For this review, take the finished solid that the model builds, in its own axes (mm). A direction names the side the tool comes from. Round coordinates to 2 decimals unless told otherwise and drop trailing zeros. Write each loop counter-clockwise with the first axis right and the second up, starting at its lowest first coordinate (ties: lowest second). Pieces come first, ordered by that corner, then holes. Notation, with made-up numbers: M 89,-37 L 94,-37 A28 cw 94,-14 Z; hole C 77,18 d7. An arc over 180 degrees is marked long. Answer in a Markdown table with one row per item.
Autodesk Inventor part; units mm, degrees
ref_plane "YZ Plane" through (0, 0, 0) normal (1, 0, 0) x (0, 1, 0)
ref_plane "XZ Plane" through (0, 0, 0) normal (0, 1, 0) x (-1, 0, 0)
ref_plane "XY Plane" through (0, 0, 0) normal (0, 0, 1) x (1, 0, 0)
sketch "Esquisse1" plane through (0, 0, 0) normal (0, 0, 1) x (1, 0, 0)
  line L0 (0, 16) -> (41, 16)
  line L1 (41, 16) -> (41, 0)
  line L2 (41, 0) -> (0, 0)
  line L3 (0, 0) -> (0, 16)
  line L4 (0, -3.2) -> (0, 19.2)
  line L5 (-8.2, 0) -> (49.2, 0)
  point P0 (0, 0)
  dimension "d0" = 16
  dimension "d1" = 41
extrude "Extrusion1" add sketch "Esquisse1" along normal blind 2
sketch "Esquisse2" plane through (0, 0, 2) normal (0, 0, 1) x (1, 0, 0)
  line L0 (1, 13) -> (3.5, 13)
  line L1 (3.5, 13) -> (3.5, 10.5)
  line L2 (3.5, 10.5) -> (1, 10.5)
  line L3 (1, 10.5) -> (1, 13)
  line L4 (3.5, 13) -> (6, 13)
  line L5 (6, 13) -> (6, 10.5)
  line L6 (6, 10.5) -> (3.5, 10.5)
  line L7 (3.5, 10.5) -> (3.5, 13)
  line L8 (0, -3.2) -> (0, 19.2)
  line L9 (1, 8) -> (1, 10.5)
  line L10 (1, 10.5) -> (3.5, 10.5)
  line L11 (3.5, 10.5) -> (3.5, 8)
  line L12 (3.5, 10.5) -> (6, 10.5)
  line L13 (6, 10.5) -> (6, 8)
  line L14 (6, 8) -> (3.5, 8)
  line L15 (3.5, 8) -> (1, 8)
  line L16 (1, 5.5) -> (1, 8)
  line L17 (1, 8) -> (3.5, 8)
  line L18 (3.5, 8) -> (3.5, 5.5)
  line L19 (3.5, 8) -> (6, 8)
  line L20 (6, 8) -> (6, 5.5)
  line L21 (6, 5.5) -> (3.5, 5.5)
  line L22 (3.5, 5.5) -> (1, 5.5)
  line L23 (1, 3) -> (1, 5.5)
  line L24 (1, 5.5) -> (3.5, 5.5)
  line L25 (3.5, 5.5) -> (3.5, 3)
  line L26 (3.5, 5.5) -> (6, 5.5)
  line L27 (6, 5.5) -> (6, 3)
  line L28 (6, 3) -> (3.5, 3)
  line L29 (3.5, 3) -> (1, 3)
  line L30 (41, 16) -> (0, 16)
  point P0 (0, 0)
  dimension "d4" = 2.5
  dimension "d5" = 2.5
  dimension "d8" = 2.5
  dimension "d9" = 2.5
  dimension "d12" = 2.5
  dimension "d17" = 3
  dimension "d18" = 1
extrude "Extrusion2" add sketch "Esquisse2" along normal blind 2
sketch "Esquisse3" plane through (0, 0, 4) normal (0, 0, 1) x (1, 0, 0)
  line L0 (1.85, 12.15) -> (2.65, 12.15)
  line L1 (2.65, 12.15) -> (2.65, 11.35)
  line L2 (2.65, 11.35) -> (1.85, 11.35)
  line L3 (1.85, 11.35) -> (1.85, 12.15)
  line L4 (6, 13) -> (1, 13)
  line L5 (1, 13) -> (1, 3)
  line L6 (2.65, 9.65) -> (2.65, 8.85)
  line L7 (1.85, 9.65) -> (2.65, 9.65)
  line L8 (1.85, 8.85) -> (1.85, 9.65)
  line L9 (2.65, 8.85) -> (1.85, 8.85)
  line L10 (2.65, 7.15) -> (2.65, 6.35)
  line L11 (1.85, 7.15) -> (2.65, 7.15)
  line L12 (1.85, 6.35) -> (1.85, 7.15)
  line L13 (2.65, 6.35) -> (1.85, 6.35)
  line L14 (2.65, 4.65) -> (2.65, 3.85)
  line L15 (1.85, 4.65) -> (2.65, 4.65)
  line L16 (1.85, 3.85) -> (1.85, 4.65)
  line L17 (2.65, 3.85) -> (1.85, 3.85)
  line L18 (5.15, 12.15) -> (5.15, 11.35)
  line L19 (4.35, 12.15) -> (5.15, 12.15)
  line L20 (4.35, 11.35) -> (4.35, 12.15)
  line L21 (5.15, 11.35) -> (4.35, 11.35)
  line L22 (5.15, 9.65) -> (5.15, 8.85)
  line L23 (4.35, 9.65) -> (5.15, 9.65)
  line L24 (4.35, 8.85) -> (4.35, 9.65)
  line L25 (5.15, 8.85) -> (4.35, 8.85)
  line L26 (5.15, 7.15) -> (5.15, 6.35)
  line L27 (4.35, 7.15) -> (5.15, 7.15)
  line L28 (4.35, 6.35) -> (4.35, 7.15)
  line L29 (5.15, 6.35) -> (4.35, 6.35)
  line L30 (5.15, 4.65) -> (5.15, 3.85)
  line L31 (4.35, 4.65) -> (5.15, 4.65)
  line L32 (4.35, 3.85) -> (4.35, 4.65)
  line L33 (5.15, 3.85) -> (4.35, 3.85)
  point P0 (0, 0)
  dimension "d21" = 0.8
  dimension "d22" = 0.8
  dimension "d23" = 0.85
  dimension "d24" = 0.85
  dimension "d27" = 2.5
  dimension "d30" = 2.5
extrude "Extrusion3" add sketch "Esquisse3" along normal blind 6
sketch "Esquisse4" plane through (0, 0, 0) normal (0, 0, -1) x (-1, 0, 0)
  line L0 (-40, 5) -> (-34, 5)
  line L1 (-34, 5) -> (-34, 11)
  line L2 (-34, 11) -> (-40, 11)
  line L3 (-40, 11) -> (-40, 5)
  line L4 (-41, 0) -> (-41, 16)
  line L5 (0, 0) -> (-41, 0)
  dimension "d35" = 6
  dimension "d36" = 6
  dimension "d37" = 1
  dimension "d38" = 5
extrude "Extrusion4" add sketch "Esquisse4" along normal blind 3
sketch "Esquisse5" plane through (0, 0, -3) normal (0, 0, -1) x (-1, 0, 0)
  circle A0 centre (-37, 8) radius 3
  line L0 (-34, 11) -> (-40, 11)
  line L1 (-40, 11) -> (-40, 5)
  line L2 (-34, 5) -> (-34, 11)
  point P0 (0, 0)
extrude "Extrusion5" add sketch "Esquisse5" along normal blind 1 contours A0
sketch "Esquisse6" plane through (37, 8, -4) normal (0, 0, -1) x (-1, 0, 0)
  line L0 (-3, -3) -> (3, -3)
  line L1 (3, -3) -> (3, 3)
  line L2 (3, 3) -> (-3, 3)
  line L3 (-3, 3) -> (-3, -3)
  line L4 (0, 3) -> (-3, 3)
  line L5 (-3, 0) -> (-3, -3)
  line L6 (-3, -3) -> (0, -3)
  line L7 (3, -3) -> (3, 0)
  point P0 (37, -8)
extrude "Extrusion6" add sketch "Esquisse6" along normal blind 7
sketch "Esquisse7" plane through (40, 8, -4) normal (1, 0, 0) x (0, 0, -1)
  circle A0 centre (4, 0) radius 3
  line L0 (7, 3) -> (7, -3)
  line L1 (0, -3) -> (7, -3)
  line L2 (0, 3) -> (7, 3)
  point P0 (-4, -8)
extrude "Extrusion7" add sketch "Esquisse7" along normal blind 9 contours A0
equation "\"d5\" = d4"
equation "\"d8\" = d4"
equation "\"d9\" = d5"
equation "\"d22\" = d21"
equation "\"d24\" = d23"
equation "\"d36\" = d35"
properties part number "nrf24"
Q1. Take a section at C-C (z = -7.25). State the section outline as (x, y) points, then the cut area to 3 significant figures.
Found:
| item | result |
|---|---|
| outline | M 34,5 L 40,5 L 40,5.1 L 49,5.1 L 49,10.9 L 40,10.9 L 40,11 L 34,11 Z |
| area | 88.3 mm² |
Q2. Take a section at A-A (z = 8). State how many separate pieces and enclosed holes the cut face has, then the cut area to 3 significant figures.
Found:
| item | result |
|---|---|
| separate pieces | 8 |
| enclosed holes | 0 |
| area | 5.12 mm² |
Q3. Mouldability with a two-part tool opening along Z and no side actions: class faces 6 (the face through (34, 8, -1)), 7 (the face through (40, 8, -1)), 8 (the face through (39.4, 10.3, -4)), 9 (the face through (37, 8, -11)) as +Z half, -Z half, draft (parallel to the pull), parting line (faces both ways), or undercut.
Found:
| item | result |
|---|---|
| face 6 | draft |
| face 7 | undercut |
| face 8 | undercut |
| face 9 | -Z half |
Q4. Take a section at B-B (y = 15). State the section outline as (x, z) points, then the cut area to 3 significant figures.
Found:
| item | result |
|---|---|
| outline | M 0,0 L 41,0 L 41,2 L 0,2 Z |
| area | 82.0 mm² |
Q5. Machinability: for faces 1 (the face through (34, 8, -7)), 2 (the face through (39.4, 5.7, -3)), 3 (the face through (37, 11, -1)), 4 (the face through (41, 8, 1)), 5 (the face through (40, 10.4, -10.3)), which of the approach directions +Z, -Z, +X, -X, +Y, -Y give a long, thin tool a straight path to every point of the face, cutting with its end or side? Answer none if there is none.
Found:
| item | result |
|---|---|
| face 1 | -Z, -X, +Y, -Y |
| face 2 | +X, -Y |
| face 3 | -Z, +X, -X, +Y |
| face 4 | +Z, +X, +Y, -Y |
| face 5 | -Z, +X, +Y |
Q6. Take a section at D-D (x = 34.5). State the section outline as (y, z) points.
Found:
| item | result |
|---|---|
| outline | M 0,0 L 5,0 L 5,-3 L 6.34,-3 L 6.34,-4 L 5,-4 L 5,-11 L 11,-11 L 11,-4 L 9.66,-4 L 9.66,-3 L 11,-3 L 11,0 L 16,0 L 16,2 L 0,2 Z |
Q7. For probe 1 along Z at (x, y) = (38.5, 15); probe 2 along X at (y, z) = (10, -2.5); probe 3 along X at (y, z) = (10.5, -9.5), list the stretches that pass through material, from the lowest coordinate up.
Found:
| item | result |
|---|---|
| probe 1 | 0 to 2 |
| probe 2 | 34 to 40 |
| probe 3 | 34 to 49 |
Q8. Insertion check: P1, Ø0.9, axis at y = 9.5, z = -2, coming from the +X side; P2, Ø1, axis at y = 7.5, z = 7.5, coming from the -X side; P3, Ø8, axis at x = 20.5, y = 10, coming from the -Z side. Each pin has a flat end and moves straight along its axis. Give the tip position at first contact, or say it passes through.
Found:
| item | result |
|---|---|
| P1 | x = 40 |
| P2 | x = 1.85 |
| P3 | z = 0 |
